Model file for the job. Use its own axes, mm. Round coordinates to 2 decimals unless told otherwise and drop trailing zeros. Order: outer loops, then holes, each group sorted by start corner. A loop starts at its lowest first (then second) coordinate and runs counter-clockwise, first axis right, second up. Notation, with made-up numbers: (78, 76.5) - (129, 76.5) arc R18 ccw to (129, 82.5) - close; hole circle Ø2 at (24.25, 50.5). An arc over 180 degrees is marked (long way). Write item = value, one per line.
```python
from build123d import *

# Parameters (mm, degrees)
SKETCH1_R           = 2.5
BOSS_EXTRUDE1_DEPTH = 2.5
SKETCH3_W           = 6
SKETCH3_H           = 6
CUT_EXTRUDE2_DEPTH  = 177.395152995
SKETCH2_R           = 1.25
CUT_EXTRUDE1_DEPTH  = 177.395152995
FILLET1_R           = 0.5
FILLET2_R           = 3


with BuildPart() as part:
    # Sketch1 → Boss-Extrude1 (new body)
    with BuildSketch(Plane.XY):
        Polygon((0, 0), (5.5, 0), (5.5, -4.5), (17.5, -4.5), (17.5, 0), (25, 0), (25, -4.5), (37, -4.5), (37, 0), (47, 0), (47, 170), (10, 170), (10, 150), (0, 150), (0, 100), (-4.5, 100), (-4.5, 75), (0, 75), (0, 50), (-4.5, 50), (-4.5, 25), (0, 25), align=None)
        with Locations((35, 5.85)):
            Circle(SKETCH1_R, mode=Mode.SUBTRACT)
        with Locations((35, 164.15)):
            Circle(SKETCH1_R, mode=Mode.SUBTRACT)
    extrude(amount=BOSS_EXTRUDE1_DEPTH)

    # Sketch3 → Cut-Extrude2 (cut, through all)
    with BuildSketch(Plane.XY.offset(2.5)):
        with Locations((44, 167)):
            Rectangle(SKETCH3_W, SKETCH3_H)
    extrude(amount=-CUT_EXTRUDE2_DEPTH, mode=Mode.SUBTRACT)

    # Sketch2 → Cut-Extrude1 (cut, through all)
    with BuildSketch(Plane.XY.offset(2.5)):
        with Locations((-0.883883476, 24.116116524)):
            Circle(SKETCH2_R)
        with Locations((-0.883883476, 50.883883476)):
            Circle(SKETCH2_R)
        with Locations((-0.883883476, 74.116116524)):
            Circle(SKETCH2_R)
        with Locations((-0.883883476, 100.883883476)):
            Circle(SKETCH2_R)
        with Locations((4.616116524, -0.883883476)):
            Circle(SKETCH2_R)
        with Locations((18.383883476, -0.883883476)):
            Circle(SKETCH2_R)
        with Locations((24.116116524, -0.883883476)):
            Circle(SKETCH2_R)
        with Locations((37.883883476, -0.883883476)):
            Circle(SKETCH2_R)
    extrude(amount=-CUT_EXTRUDE1_DEPTH, mode=Mode.SUBTRACT)

    # Fillet1
    fillet1_edges = [part.edges().sort_by_distance(p)[0] for p in [
        (-4.5, 25, 1.25),
        (-4.5, 50, 1.25),
        (-4.5, 75, 1.25),
        (-4.5, 100, 1.25),
        (0, 150, 1.25),
        (10, 170, 1.25),
        (47, 0, 1.25),
        (37, -4.5, 1.25),
        (25, -4.5, 1.25),
        (17.5, -4.5, 1.25),
        (5.5, -4.5, 1.25),
        (41, 170, 1.25),
        (47, 164, 1.25),
    ]]
    fillet(fillet1_edges, radius=FILLET1_R)

    # Fillet2
    fillet2_edges = [part.edges().sort_by_distance(p)[0] for p in [
        (10, 150, 1.25),
        (41, 164, 1.25),
    ]]
    fillet(fillet2_edges, radius=FILLET2_R)


solid = part.part
```
1) Cut at B-B (x = 35). Write the cut outline in (y, z), and give its area (3 significant figures).
Conclusion:
outline = (-4.5, 0) - (3.35, 0) - (3.35, 2.5) - (-4.5, 2.5) - close; (8.35, 0) - (161.65, 0) - (161.65, 2.5) - (8.35, 2.5) - close; (166.65, 0) - (170, 0) - (170, 2.5) - (166.65, 2.5) - close
area = 411 mm^2
2) Cut at D-D (y = 157). Write the cut outline in (x, z).
Conclusion:
outline = (10, 0) - (47, 0) - (47, 2.5) - (10, 2.5) - close
3) Wall check: line 1 along Y through (x, z) = (1, 0.75); line 2 along X through (y, z) = (11, 2.35); line 3 along Y through (x, z) = (-1.5, 0.35). Give the ranges that are in metal, low to high.
Conclusion:
line_1 = 0 to 150
line_2 = 0 to 47
line_3 = 25.2 to 49.8, 75.2 to 99.8
4) Mould opens along Y. For faces 1 (the face through (21, 84, 0)), 2 (the face through (37.385, 6.601, 1.232)), 3 (the face through (9.1, 150.86, 1.27)) say: +Y half, -Y half, draft (parallel to the pull), parting line (faces both ways), or undercut.
Conclusion:
face_1 = draft
face_2 = undercut
face_3 = +Y half
5) Cut at A-A (y = 5.85). Write the cut outline in (x, z), and give its area (3 significant figures).
Conclusion:
outline = (0, 0) - (32.5, 0) - (32.5, 2.5) - (0, 2.5) - close; (37.5, 0) - (47, 0) - (47, 2.5) - (37.5, 2.5) - close
area = 105 mm^2
6) Flat gauge pins, fed straight in: pin 1 Ø1.2 at (y, z) = (158, 2) entering from -X; pin 2 Ø1.2 at (x, z) = (46, 1) entering from +Y; pin 3 Ø1.1 at (y, z) = (-3, 1.5) entering from +X. Where does each tip first touch, or does it go through?
Conclusion:
pin_1 = 10
pin_2 = 164
pin_3 = 37
7) Cut at C-C (z = 1.75). Give the number of separate pieces and of enclosed holes in the cut face, and give its area (3 significant figures).
Conclusion:
separate_pieces = 1
enclosed_holes = 2
area = 8,040 mm^2
